Geometry: final body of the model. Coordinates: model frame, mm. Face numbers are marked on the shaded views. Give positions to 0.01 mm unless a question says otherwise; leave off trailing zeros. Loops run counter-clockwise (first coordinate to the right, second up) from the corner with the lowest first, then second, coordinate; pieces in that order, holes last. Notation, with made-up numbers: (28, -38) - (36, -38) arc R23 ccw to (36, -19) - close; hole circle Ø1 at (-22.75, 62.25). An arc over 180 degrees is marked (long way). Use one line per item in the form item = value.
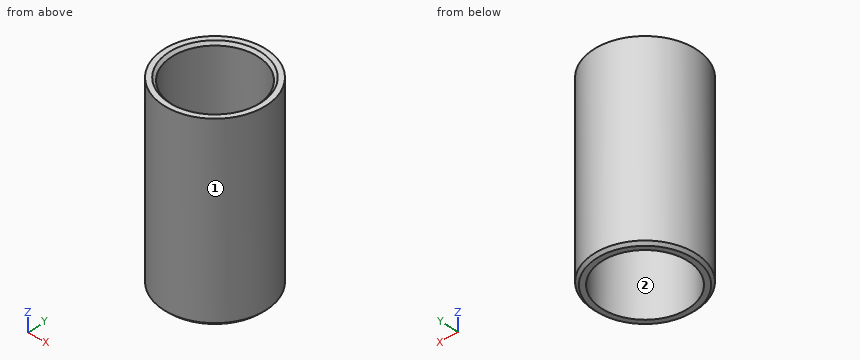
```python
from build123d import *

# Parameters (mm, degrees)
F0_R     = 18.5
F1_DEPTH = 68
F2_R     = 15.6
F3_DEPTH = 68.001
F4_SIZE  = 1
F5_SIZE  = 1


with BuildPart() as f1:
    # F0 (on Top) → F1 (new body)
    with BuildSketch(Plane.XY):
        Circle(F0_R)
    extrude(amount=F1_DEPTH)

    # F2 (on Top) → F3 (cut, through all)
    with BuildSketch(Plane.XY):
        Circle(F2_R)
    extrude(amount=F3_DEPTH, mode=Mode.SUBTRACT)

    # F4
    f4_edges = [f1.edges().sort_by_distance(p)[0] for p in [
        (-18.5, 0, 0),
    ]]
    chamfer(f4_edges, length=F4_SIZE)

    # F5
    f5_edges = [f1.edges().sort_by_distance(p)[0] for p in [
        (-15.6, 0, 68),
    ]]
    chamfer(f5_edges, length=F5_SIZE)


solid = f1.part
```
(1) Pull-direction query (Y, two-part tool) for the marked faces 1 and 2; classes: released by +Y, released by -Y, zero draft, split by the parting line, or undercut.
Solution:
face_1 = split by the parting line
face_2 = undercut
(2) Material intervals for L1, parallel to Y at x = 0, z = 48; L2, parallel to X at y = -3, z = 41.5; L3, parallel to X at y = 2, z = 47.5, sorted ascending. Write a range as from..to.
Solution:
L1 = -18.5..-15.6, 15.6..18.5
L2 = -18.26..-15.31, 15.31..18.26
L3 = -18.39..-15.47, 15.47..18.39
(3) Cut plane A-A (x = 0). Return the cut outline in (y, z).
Solution:
outline = (-18.5, 1) - (-17.5, 0) - (-15.6, 0) - (-15.6, 67) - (-16.6, 68) - (-18.5, 68) - close; (15.6, 0) - (17.5, 0) - (18.5, 1) - (18.5, 68) - (16.6, 68) - (15.6, 67) - close
(4) Cut plane C-C (z = 11). Return the cut outline in (x, y), plus the area to 3 significant figures.
Solution:
outline = circle Ø37 at (0, 0); hole circle Ø31.2 at (0, 0)
area = 311 mm2
(5) Pin query (flat end, axial travel): P1, Ø1, axis at y = 13.5, z = 28.5, coming from the -X side; P2, Ø12, axis at x = 4, z = 34, coming from the +Y side; P3, Ø2, axis at x = -14, z = 36, coming from the +Y side. Return the tip coordinate at first contact, or that it passes through.
Solution:
P1 = -13.16
P2 = 18.5
P3 = 13.16
